Could you check a few things on this model? Use its own coordinates, in mm. Coordinates: 2 decimals unless noted, no trailing zeros. Loops run counter-clockwise (first coordinate to the right, second up) from the corner with the lowest first, then second, coordinate; pieces in that order, holes last.
1) Imagine slicing it at A-A on z = 0. Please give me the cut outline in (x, y).
2) Imagine slicing it at B-B on y = 8. Please give me the cut outline in (x, z), plus the area to 3 significant figures.
3) If I drill on line 1 along X through (y, z) = (6.5, 0); line 2 along X through (y, z) = (13.5, -1.2); line 3 along Z through (x, y) = (1.15, 1.5), over which ranges is the centre line in solid material (lowest first)?
4) Thinking about a two-plate mould opening in X: for faces 1 (the face through (-0.07, 7.4, 1.75)), 2 (the face through (0, 0, 2)), 3 (the face through (0.1, 14.86, 2.54)), which applies, released by +X, released by -X, zero draft, split by the parting line, or undercut?
5) Will these pins go through, and if not, where does the flat tip stop? P1, Ø0.6, axis at y = 4.5, z = -2, coming from the -X side; P2, Ø3, axis at x = -2, y = 9.5, coming from the -Z side; P3, Ø2, axis at x = 0, z = 0, coming from the -Y side.
6) Imagine slicing it at C-C on x = 0. Please give me the cut outline in (y, z), plus the area to 3 significant figures.
```python
from build123d import *
from OCP.BRepFilletAPI import BRepFilletAPI_MakeChamfer

# Parameters (mm, degrees)
ESBO_O1_R                = 2.75
ESBO_O1_R_2              = 1.75
RESSALTO_EXTRUS_O1_DEPTH = 15
ESBO_O2_W                = 1.5
ESBO_O2_H                = 2.767894019
CORTE_EXTRUS_O1_DEPTH    = 16.495967217
CHANFRO1_SIZE            = 0.5
CHANFRO2_SIZE            = 0.5
CHANFRO2_SIZE2           = 0.288675135


with BuildPart() as part:
    # Esboço1 → Ressalto-extrusão1 (new body)
    with BuildSketch(Plane(origin=(0, 0, 0), x_dir=(1, 0, 0), z_dir=(0, 1, 0))):
        with Locations(Location((0, 0, 0), (0, 0, 270))):
            Circle(ESBO_O1_R)
        with Locations(Location((0, 0, 0), (0, 0, 270))):
            Circle(ESBO_O1_R_2, mode=Mode.SUBTRACT)
    extrude(amount=RESSALTO_EXTRUS_O1_DEPTH)

    # Esboço2 → Corte-extrusão1 (cut, through all)
    with BuildSketch(Plane(origin=(0, 15, 0), x_dir=(1, 0, 0), z_dir=(0, 1, 0))):
        with Locations((0, 1.747513295)):
            Rectangle(ESBO_O2_W, ESBO_O2_H)
    extrude(amount=-CORTE_EXTRUS_O1_DEPTH, mode=Mode.SUBTRACT)

    # Chanfro1
    # the kernel refuses this chamfer: 0.5, 0.257849129 mm, written as the material it takes off along each edge
    with BuildSketch(Plane(origin=(-0.75, 16.293542877, -2.645751311), x_dir=(-0.9484043695289113, 0, 0.3170633246821023), z_dir=(0, -1, 0))) as chanfro1_piece_1:
        with BuildLine():
            Line((0.25513486, 0), (CHANFRO1_SIZE * 0.317063324682, -CHANFRO1_SIZE * 0.948404369529))
            Line((CHANFRO1_SIZE * 0.317063324682, -CHANFRO1_SIZE * 0.948404369529), (0, 0))
            ThreePointArc((0, 0), (0.129558651, 0.002959681), (0.25513486, 0))
        make_face()
    extrude(amount=17.587085755, mode=Mode.SUBTRACT)
    with BuildSketch(Plane(origin=(0.75, 16.293542877, -2.645751311), x_dir=(0.948404369528912, 0, 0.3170633246821001), z_dir=(0, -1, 0))) as chanfro1_piece_2:
        with BuildLine():
            Line((0.25513486, 0), (CHANFRO1_SIZE * 0.317063324682, CHANFRO1_SIZE * 0.948404369529))
            Line((CHANFRO1_SIZE * 0.317063324682, CHANFRO1_SIZE * 0.948404369529), (0, 0))
            ThreePointArc((0, 0), (0.129558651, -0.002959681), (0.25513486, 0))
        make_face()
    extrude(amount=17.587085755, mode=Mode.SUBTRACT)

    # Chanfro2: one chamfer whose edges measure the first distance from different faces: ONE call of the kernel's chamfer builder (chamfer() names one face for all edges)
    chanfro2_edges_1 = [part.edges().sort_by_distance(p)[0] for p in [
        (0, 0, 2.75),
    ]]
    chanfro2_side_1 = [part.faces().sort_by_distance(p)[0] for p in [
        (-0.937222417, 0, -2.31706246),
    ]]
    chanfro2_edges_2 = [part.edges().sort_by_distance(p)[0] for p in [
        (0, 15, 2.75),
    ]]
    chanfro2_side_2 = [part.faces().sort_by_distance(p)[0] for p in [
        (0, 7.5, 2.75),
    ]]
    chanfro2 = BRepFilletAPI_MakeChamfer(part.part.solid().wrapped)
    for e in chanfro2_edges_1:
        chanfro2.Add(CHANFRO2_SIZE, CHANFRO2_SIZE2, e.wrapped, chanfro2_side_1[0].wrapped)  # the first distance lies on this face
    for e in chanfro2_edges_2:
        chanfro2.Add(CHANFRO2_SIZE, CHANFRO2_SIZE2, e.wrapped, chanfro2_side_2[0].wrapped)  # the first distance lies on this face
    add(Compound.cast(chanfro2.Shape()), mode=Mode.REPLACE)


solid = part.part
```
Filled in:
1. outline: (-2.75, 0.29) - (-2.25, 0) - (-1.75, 0) - (-1.75, 15) - (-2.46, 15) - (-2.75, 14.5) - close; (1.75, 0) - (2.25, 0) - (2.75, 0.29) - (2.75, 14.5) - (2.46, 15) - (1.75, 15) - close
2. outline: (-0.99, -2.56) - (-0.75, -2.15) - (-0.75, -1.58) arc R1.75 cw (long way) to (0.75, -1.58) - (0.75, -2.15) - (0.99, -2.56) arc R2.75 ccw (long way) to start
2. area: 12.5 mm2
3. line 1: x = -2.75 to -1.75, 1.75 to 2.75
3. line 2: x = -2.47 to -1.27, 1.27 to 2.47
3. line 3: z = -2.5 to -1.32, 1.32 to 2.5
4. face 1: undercut
4. face 2: zero draft
4. face 3: split by the parting line
5. P1: stops at x = -2.16
5. P2: stops at z = -2.56
5. P3: passes through
6. outline: (0, 1.75) - (15, 1.75) - (15, 2.46) - (14.5, 2.75) - (0.29, 2.75) - (0, 2.25) - close
6. area: 14.9 mm2
